Work out the finished part from the listing and answer in its coordinate system (mm). Face numbers are marked on the shaded views. A direction names the side the tool comes from. Coordinates: 2 decimals unless noted, no trailing zeros. Write each loop counter-clockwise with the first axis right and the second up, starting at its lowest first coordinate (ties: lowest second). Pieces come first, ordered by that corner, then holes. Notation, with made-up numbers: (42, 68.5) - (89, 68.5) arc R27 ccw to (89, 91.5) - close; hole circle Ø11 at (44.25, 57). An arc over 180 degrees is marked (long way). Use a Markdown table: item, result. Add a question column.
(1) The part is cut by section D-D, the plane x = -9.5. Give the vertices of the cut face in (y, z), then the cut area to 3 significant figures.
(2) Find the intervals of material crossed by line 1 (Y direction, x = 9.5, z = 3.8); line 2 (X direction, y = 2.25, z = 4.5); line 3 (X direction, y = 5.5, z = 0.25), in increasing order. Write a range as from..to.
(3) For a pull along X with two mould halves and no side action, classify the marked faces 1, 2, 3 and 4 as released by +X, released by -X, zero draft, split by the parting line, or undercut.
(4) The part is cut by section B-B, the plane z = 3. Give the vertices of the cut face in (x, y), then the cut area to 3 significant figures.
(5) The part is cut by section A-A, the plane y = 3. Give the vertices of the cut face in (x, z), then the cut area to 3 significant figures.
(6) The part is cut by section C-C, the plane z = 5. Give the vertices of the cut face in (x, y).
(7) Given pin 1 Ø3 at (x, y) = (-9.5, 3.5) entering from -Z; pin 2 Ø2 at (y, z) = (2, 0.5) entering from -X; pin 3 Ø1.5 at (x, y) = (0, 2) entering from +Z, each flat-ended and moving along its own axis, determine where each tip first touches the part or whether it passes through.
(8) A tool of negligible diameter and unlimited length cuts with its end or side. For the marked faces 5, 6 and 7, from which of +Z, -Z, +X, -X, +Y, -Y can it reach the whole face along a straight path? Write none if from no direction.
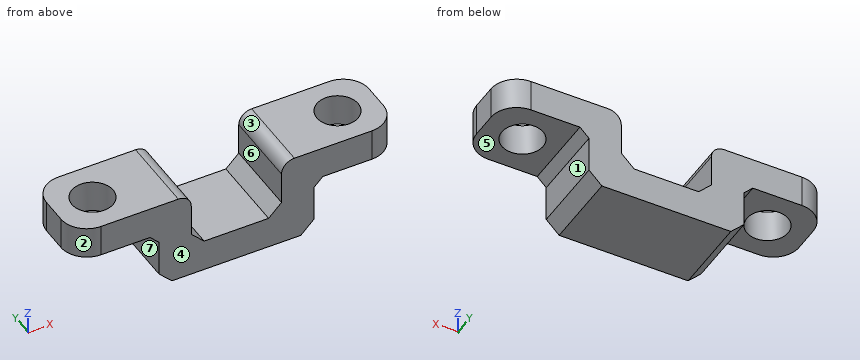
from build123d import *

# Parameters (mm, degrees)
SKETCH2_W           = 6.5
SKETCH2_H           = 2.5
SKETCH2_W_2         = 7
BOSS_EXTRUDE2_DEPTH = 6
SKETCH3_R           = 1.6
CUT_EXTRUDE1_DEPTH  = 3.5
CHAMFER1_SIZE       = 1
FILLET1_R           = 2
FILLET2_R           = 1
CHAMFER2_SIZE       = 0.7


with BuildPart() as part:
    # Sketch2 → Boss-Extrude2 (new body)
    with BuildSketch(Plane(origin=(0, 0, 0), x_dir=(1, 0, 0), z_dir=(0, 1, 0))):
        with Locations((-9.25, -4.5)):
            Rectangle(SKETCH2_W, SKETCH2_H)
        Polygon((-3.5, -5.75), (-3.5, -1.25), (-3.5, 1.25), (-6, 1.25), (-6, -3.25), (-6, -5.75), align=None)
        Rectangle(SKETCH2_W_2, SKETCH2_H)
        Polygon((3.5, 1.25), (3.5, -1.25), (3.5, -5.75), (6, -5.75), (6, -3.25), (6, 1.25), align=None)
        with Locations((9.25, -4.5)):
            Rectangle(SKETCH2_W, SKETCH2_H)
    extrude(amount=BOSS_EXTRUDE2_DEPTH)

    # Sketch3 → Cut-Extrude1 (cut, through all)
    with BuildSketch(Plane(origin=(0, 0, 3.25), x_dir=(-1, 0, 0), z_dir=(0, 0, -1))):
        with Locations((-9.5, 3)):
            Circle(SKETCH3_R)
        with Locations((9.5, 3)):
            Circle(SKETCH3_R)
    extrude(amount=-CUT_EXTRUDE1_DEPTH, mode=Mode.SUBTRACT)

    # Chamfer1
    chamfer1_edges = [part.edges().sort_by_distance(p)[0] for p in [
        (-6, 3, -1.25),
        (6, 3, -1.25),
        (3.5, 3, 1.25),
        (-3.5, 3, 1.25),
    ]]
    chamfer(chamfer1_edges, length=CHAMFER1_SIZE)

    # Fillet1
    fillet1_edges = [part.edges().sort_by_distance(p)[0] for p in [
        (12.5, 0, 4.5),
        (-12.5, 0, 4.5),
        (12.5, 6, 4.5),
        (-12.5, 6, 4.5),
    ]]
    fillet(fillet1_edges, radius=FILLET1_R)

    # Fillet2
    fillet2_edges = [part.edges().sort_by_distance(p)[0] for p in [
        (3.5, 3, 5.75),
        (-3.5, 3, 5.75),
    ]]
    fillet(fillet2_edges, radius=FILLET2_R)

    # Chamfer2
    chamfer2_edges = [part.edges().sort_by_distance(p)[0] for p in [
        (-6, 3, 3.25),
        (6, 3, 3.25),
    ]]
    chamfer(chamfer2_edges, length=CHAMFER2_SIZE)


solid = part.part
Model answer:
| question | item | result |
|---|---|---|
| 1 | outline | (0, 3.25) - (1.4, 3.25) - (1.4, 5.75) - (0, 5.75) - close; (4.6, 3.25) - (6, 3.25) - (6, 5.75) - (4.6, 5.75) - close |
| 1 | area | 7.00 mm^2 |
| 2 | line 1 | 0..1.4, 4.6..6 |
| 2 | line 2 | -12.5..-10.91, -8.09..-3.5, 3.5..8.09, 10.91..12.5 |
| 2 | line 3 | -6..6 |
| 3 | face 1 | released by +X |
| 3 | face 2 | released by -X |
| 3 | face 3 | undercut |
| 3 | face 4 | zero draft |
| 4 | outline | (-6.45, 0) - (-3.5, 0) - (-3.5, 6) - (-6.45, 6) - close; (3.5, 0) - (6.45, 0) - (6.45, 6) - (3.5, 6) - close |
| 4 | area | 35.4 mm^2 |
| 5 | outline | (-12.5, 3.25) - (-11.1, 3.25) - (-11.1, 5.75) - (-12.5, 5.75) - close; (-7.9, 3.25) - (-6.7, 3.25) - (-6, 2.55) - (-6, -0.25) - (-5, -1.25) - (5, -1.25) - (6, -0.25) - (6, 2.55) - (6.7, 3.25) - (7.9, 3.25) - (7.9, 5.75) - (4.5, 5.75) arc R1 ccw to (3.5, 4.75) - (3.5, 2.25) - (2.5, 1.25) - (-2.5, 1.25) - (-3.5, 2.25) - (-3.5, 4.75) arc R1 ccw to (-4.5, 5.75) - (-7.9, 5.75) - close; (11.1, 3.25) - (12.5, 3.25) - (12.5, 5.75) - (11.1, 5.75) - close |
| 5 | area | 69.1 mm^2 |
| 6 | outline | (-12.5, 2) arc R2 ccw to (-10.5, 0) - (-3.53, 0) - (-3.53, 6) - (-10.5, 6) arc R2 ccw to (-12.5, 4) - close; (3.53, 0) - (10.5, 0) arc R2 ccw to (12.5, 2) - (12.5, 4) arc R2 ccw to (10.5, 6) - (3.53, 6) - close; hole circle Ø3.2 at (-9.5, 3); hole circle Ø3.2 at (9.5, 3) |
| 7 | pin 1 | z = 3.25 |
| 7 | pin 2 | x = -6 |
| 7 | pin 3 | z = 1.25 |
| 8 | face 5 | -Z, +X, +Y, -Y |
| 8 | face 6 | +Z, +Y, -Y |
| 8 | face 7 | -Z, -X, +Y, -Y |
